from build123d import *

# Parameters (mm, degrees)
SKETCH1_R                = 40
SKETCH1_R_2              = 34
BOSS_EXTRUDE1_DEPTH      = 15
SKETCH1_3_R              = 34
BOSS_EXTRUDE2_DEPTH      = 16
SKETCH1_4_R              = 34
SKETCH1_4_R_2            = 29
BOSS_EXTRUDE3_DEPTH      = 2
BOSS_EXTRUDE4_DEPTH      = 5
BOSS_EXTRUDE4_DEPTH_BACK = 5
SKETCH2_R                = 2.25
CUT_EXTRUDE1_DEPTH       = 10
BOSS_EXTRUDE5_START      = -10
BOSS_EXTRUDE5_DEPTH      = 3
SKETCH4_R                = 2.25
CUT_EXTRUDE3_DEPTH       = 3


with BuildPart() as part:
    # Sketch1 → Boss-Extrude1 (new body)
    with BuildSketch(Plane(origin=(0, 0, 0), x_dir=(1, 0, 0), z_dir=(0, 1, 0))):
        Circle(SKETCH1_R)
        Circle(SKETCH1_R_2, mode=Mode.SUBTRACT)
    extrude(amount=BOSS_EXTRUDE1_DEPTH)

    # Sketch1<3> → Boss-Extrude2 (add)
    with BuildSketch(Plane(origin=(0, 0, 0), x_dir=(1, 0, 0), z_dir=(0, 1, 0))):
        with BuildLine():
            ThreePointArc((19.364916731, 35), (0, 40), (-19.364916731, 35))
            ThreePointArc((-19.364916731, 35), (-20.315060063, -34.457195687), (40, 0))
            ThreePointArc((40, 0), (34.457195687, 20.315060063), (19.364916731, 35))
        make_face()
        Circle(SKETCH1_3_R, mode=Mode.SUBTRACT)
    extrude(amount=-BOSS_EXTRUDE2_DEPTH)

    # Sketch1<4> → Boss-Extrude3 (add)
    with BuildSketch(Plane(origin=(0, 0, 0), x_dir=(1, 0, 0), z_dir=(0, 1, 0))):
        Circle(SKETCH1_4_R)
        Circle(SKETCH1_4_R_2, mode=Mode.SUBTRACT)
    extrude(amount=-BOSS_EXTRUDE3_DEPTH)

    # Sketch1<5> → Boss-Extrude4 (add, two sides)
    with BuildSketch(Plane(origin=(0, 0, 0), x_dir=(1, 0, 0), z_dir=(0, 1, 0))) as boss_extrude4_sk:
        with BuildLine():
            Line((-19.364916731, 35), (-27.080992435, 35))
            Line((-27.080992435, 35), (-77.920992435, 35))
            Line((-77.920992435, 35), (-87.920992435, 35))
            Line((-87.920992435, 35), (-87.920992435, -65))
            Line((-87.920992435, -65), (-77.920992435, -65))
            Line((-77.920992435, -65), (0, -65))
            Line((0, -65), (72.08, -65))
            Line((72.08, -65), (72.08, 35))
            Line((72.08, 35), (37.080992435, 35))
            Line((37.080992435, 35), (19.364916731, 35))
            ThreePointArc((19.364916731, 35), (34.457195687, 20.315060063), (40, 0))
            ThreePointArc((40, 0), (-20.315060063, -34.457195687), (-19.364916731, 35))
        make_face()
    extrude(amount=BOSS_EXTRUDE4_DEPTH)
    extrude(boss_extrude4_sk.sketch, amount=-BOSS_EXTRUDE4_DEPTH_BACK)

    # Sketch2 → Cut-Extrude1 (cut)
    with BuildSketch(Plane.XY.offset(65)):
        with Locations((-77.920992435, 0)):
            Circle(SKETCH2_R)
        with Locations((-7.920496218, 0)):
            Circle(SKETCH2_R)
        with Locations((62.08, 0)):
            Circle(SKETCH2_R)
    extrude(amount=-CUT_EXTRUDE1_DEPTH, mode=Mode.SUBTRACT)

    # Sketch3 → Boss-Extrude5 (add)
    with BuildSketch(Plane(origin=(0, 5, 0), x_dir=(1, 0, 0), z_dir=(0, 1, 0)).offset(BOSS_EXTRUDE5_START)):
        with BuildLine():
            Line((19.364916731, 35), (62.079007565, 35))
            Line((62.079007565, 35), (72.08, 35))
            Line((72.08, 35), (72.08, -75))
            Line((72.08, -75), (62.079007565, -75))
            Line((62.079007565, -75), (-77.920992435, -75))
            Line((-77.920992435, -75), (-87.920992435, -75))
            Line((-87.920992435, -75), (-87.920992435, 35))
            Line((-87.920992435, 35), (-19.364916731, 35))
            ThreePointArc((-19.364916731, 35), (0, -40), (19.364916731, 35))
        make_face()
    extrude(amount=-BOSS_EXTRUDE5_DEPTH)

    # Sketch4 → Cut-Extrude3 (cut)
    with BuildSketch(Plane(origin=(0, -5, 0), x_dir=(-1, 0, 0), z_dir=(0, 1, 0))):
        with Locations((52.920992435, 70)):
            Circle(SKETCH4_R)
        with Locations((-37.08, 70)):
            Circle(SKETCH4_R)
    extrude(amount=-CUT_EXTRUDE3_DEPTH, mode=Mode.SUBTRACT)


solid = part.part
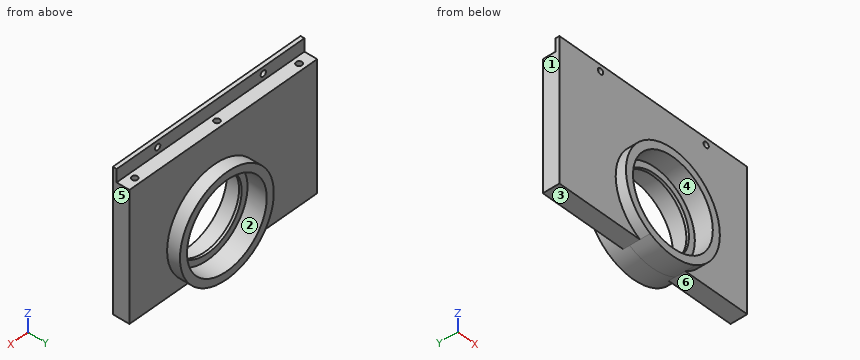
Read the model definition and answer for the solid it produces. Units are mm, in the model's axes. Face numbers are marked on the shaded views. A direction names the side the tool comes from. Round coordinates to 2 decimals unless told otherwise and drop trailing zeros. Loops run counter-clockwise (first coordinate to the right, second up) from the corner with the lowest first, then second, coordinate; pieces in that order, holes last. Notation, with made-up numbers: (81, 16.5) - (128, 16.5) arc R10 ccw to (128, 21.5) - close; hole circle Ø9 at (-24.5, 31). An arc over 180 degrees is marked (long way). One line per question, with ' | ' between items. Start each with the question number.
Q1. Find the intervals of material crossed by L1, parallel to Y at x = -60, z = 8.5; L2, parallel to Z at x = 40, y = -1.5; L3, parallel to X at y = 9.5, z = 15, in increasing order.
Q2. Section A-A on x = 0 is taken. Give the vertices of the cut face in (y, z).
Q3. Section D-D on z = 14 is taken. Give the vertices of the cut face in (x, y).
Q4. Section B-B on x = 62.08 is taken. Give the vertices of the cut face in (y, z), plus the area to 4 significant figures.
Q5. For the marked faces 4, 5 and 6, determine the directions among +Z, -Z, +X, -X, +Y, -Y from which every point of the face is accessible in a straight line to the end or side of a thin tool.
Q6. Section C-C on y = -14 is taken. Give the vertices of the cut face in (x, z).
Q7. Flat-ended cylindrical pins translate along their axes: pin 1 (11 mm diameter, centred on x = -24.5, y = 1, fed in from +Z); pin 2 (7 mm diameter, centred on x = -7.92, y = 0, fed in from -Z); pin 3 (2.5 mm diameter, centred on x = -52.92, z = 70, fed in from +Y); pin 4 (1.5 mm diameter, centred on x = 23.5, z = 22.5, fed in from +Y). Find the tip coordinate at first contact, or state that the pin passes through.
Q8. For a pull along Z with two mould halves and no side action, classify the marked faces 1, 2 and 3 as +Z half, -Z half, draft (parallel to the pull), parting line (faces both ways), or undercut.
Established:
1) L1: -8 to 5 | L2: -35 to 65 | L3: -37.08 to -30.51, 30.51 to 37.08
2) outline: (-16, -40) - (15, -40) - (15, -34) - (0, -34) - (0, -29) - (-2, -29) - (-2, -34) - (-16, -34) - close; (-16, 34) - (-2, 34) - (-2, 29) - (0, 29) - (0, 34) - (15, 34) - (15, 40) - (5, 40) - (5, 65) - (-5, 65) - (-5, 75) - (-8, 75) - (-8, 40) - (-16, 40) - close
3) outline: (-87.92, -8) - (-37.47, -8) - (-37.47, -16) - (-30.98, -16) - (-30.98, -2) - (-25.4, -2) - (-25.4, 0) - (-30.98, 0) - (-30.98, 15) - (-37.47, 15) - (-37.47, 5) - (-87.92, 5) - close; (25.4, -2) - (30.98, -2) - (30.98, -16) - (37.47, -16) - (37.47, -8) - (72.08, -8) - (72.08, 5) - (37.47, 5) - (37.47, 15) - (30.98, 15) - (30.98, 0) - (25.4, 0) - close
4) outline: (-8, -35) - (5, -35) - (5, 65) - (2.25, 65) - (2.25, 55) - (-2.25, 55) - (-2.25, 65) - (-5, 65) - (-5, 75) - (-8, 75) - close | area: 1,285 mm²
5) face 4: -Y | face 5: +Z, -Z, +X, +Y, -Y | face 6: -Z, +X, +Y, -Y
6) outline: circle Ø80 at (0, 0); hole circle Ø68 at (0, 0)
7) pin 1: z = 65 | pin 2: z = -39.76 | pin 3: through | pin 4: y = 0
8) face 1: draft | face 2: undercut | face 3: -Z half
